```python
from build123d import *

# Parameters (mm, degrees)
F0_R     = 6.5
F1_DEPTH = 3
F2_R     = 4.9
F3_DEPTH = 10
F4_R     = 1


with BuildPart() as f1:
    # F0 (on Top) → F1 (new body)
    with BuildSketch(Plane.XY):
        Circle(F0_R)
    extrude(amount=F1_DEPTH)

    # F2 (on Top) → F3 (join)
    with BuildSketch(Plane.XY):
        Circle(F2_R)
    extrude(amount=F3_DEPTH)

    # F4
    f4_edges = [f1.edges().sort_by_distance(p)[0] for p in [
        (-4.9, 0, 10),
    ]]
    fillet(f4_edges, radius=F4_R)


solid = f1.part
```
CAD build for the part. Positions are in the model's coordinates, mm. A direction names the side the tool comes from. Coordinates: 2 decimals unless noted, no trailing zeros. Write each loop counter-clockwise with the first axis right and the second up, starting at its lowest first coordinate (ties: lowest second). Pieces come first, ordered by that corner, then holes.
(1) 3-axis set-ups, long thin cutter, end or side, ignore diameter. For faces 1 (the face through (-1.062, -4.783, 5.958)), 2 (the face through (0, 0, 0)): which of +Z, -Z, +X, -X, +Y, -Y reach the whole face in a straight line?
(2) Drill centre lines: probe 1 along Z at (x, y) = (0, 6); probe 2 along Y at (x, z) = (-4.25, 2.75); probe 3 along X at (y, z) = (-4.5, 6.5). Where is each one in solid material? Low to high.
(3) Flat gauge pins, fed straight in: pin 1 (1.5 mm diameter, centred on x = 0, z = 6, fed in from +Y); pin 2 (5 mm diameter, centred on y = -5, z = 4.5, fed in from +X); pin 3 (5 mm diameter, centred on y = -0.5, z = 6.5, fed in from -X). Where does each tip first touch, or does it go through?
(4) Cut at A-A, the plane y = 0. List the corners of the cut face in (x, z).
(5) Cut at C-C, the plane z = 8.25. List the corners of the cut face in (x, y), and give its area (3 significant figures).
Geometry says:
1. face 1: +Z
1. face 2: -Z, +X, -X, +Y, -Y
2. probe 1: z = 0 to 3
2. probe 2: y = -4.92 to 4.92
2. probe 3: x = -1.94 to 1.94
3. pin 1: stops at y = 4.9
3. pin 2: stops at x = 5.77
3. pin 3: stops at x = -4.9
4. outline: (-6.5, 0) - (6.5, 0) - (6.5, 3) - (4.9, 3) - (4.9, 9) arc R1 ccw to (3.9, 10) - (-3.9, 10) arc R1 ccw to (-4.9, 9) - (-4.9, 3) - (-6.5, 3) - close
5. outline: circle Ø9.8 at (0, 0)
5. area: 75.4 mm2
